```python
from build123d import *

# Parameters (mm, degrees)
BOSS_EXTRUDE1_DEPTH     = 5
CUT_EXTRUDE1_DEPTH      = 57
CUT_EXTRUDE1_DEPTH_BACK = 57
SKETCH2_R               = 3


with BuildPart() as part:
    # Sketch1 → Boss-Extrude1 (new body)
    with BuildSketch(Plane(origin=(0, 0, 0), x_dir=(1, 0, 0), z_dir=(0, 1, 0))):
        Polygon((0, -45), (21, -45), (21, -21), (45, -21), (45, 0), (295, 0), (295, -21), (319, -21), (319, -45), (340, -45), (340, -295), (319, -295), (319, -319), (295, -319), (295, -340), (45, -340), (45, -319), (21, -319), (21, -295), (0, -295), align=None)
    extrude(amount=BOSS_EXTRUDE1_DEPTH)

    # Sketch2 → Cut-Extrude1 (cut, two sides: drawn at the far end of the back side and taken through both)
    with BuildSketch(Plane(origin=(0, 5, 0), x_dir=(1, 0, 0), z_dir=(0, 1, 0)).offset(-CUT_EXTRUDE1_DEPTH_BACK)):
        with Locations(Location((100, -10, 0), (0, 0, 270))):
            Circle(SKETCH2_R)
        with Locations(Location((240, -10, 0), (0, 0, 270))):
            Circle(SKETCH2_R)
        with Locations(Location((240, -330, 0), (0, 0, 270))):
            Circle(SKETCH2_R)
        with Locations(Location((100, -330, 0), (0, 0, 270))):
            Circle(SKETCH2_R)
        with Locations(Location((10, -240, 0), (0, 0, 270))):
            Circle(SKETCH2_R)
        with Locations(Location((10, -100, 0), (0, 0, 270))):
            Circle(SKETCH2_R)
        with Locations(Location((330, -240, 0), (0, 0, 270))):
            Circle(SKETCH2_R)
        with Locations(Location((330, -100, 0), (0, 0, 270))):
            Circle(SKETCH2_R)
    extrude(amount=CUT_EXTRUDE1_DEPTH + CUT_EXTRUDE1_DEPTH_BACK, mode=Mode.SUBTRACT)


solid = part.part
```
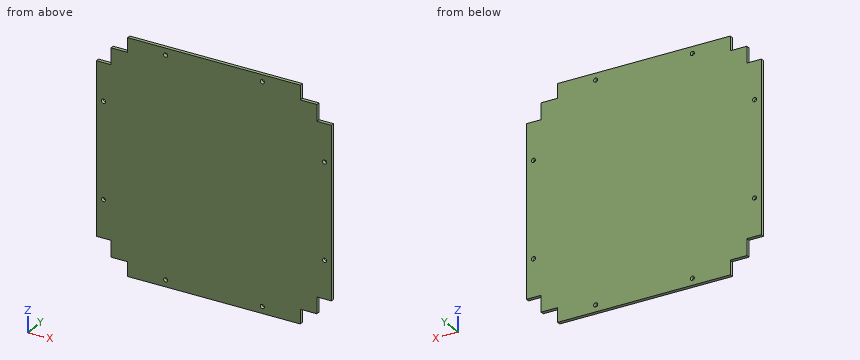
Source: CAD feature listing. Evaluate the final solid. Frame: model axes, mm. Round coordinates to 2 decimals unless told otherwise and drop trailing zeros. Write each loop counter-clockwise with the first axis right and the second up, starting at its lowest first coordinate (ties: lowest second). Pieces come first, ordered by that corner, then holes. Notation, with made-up numbers: M 1.25,0.25 L 43.25,0.25 A4 cw 43.25,7.25 Z; hole C 81,67 d10. An arc over 180 degrees is marked long. Answer as a JSON object with one key per item and string values. Group by question number.
(1) First-contact query: pin 1 (2.5 mm diameter, centred on x = 32, y = 3, fed in from +Z); pin 2 (2.5 mm diameter, centred on y = 3, z = 330, fed in from +X). Flat tips, straight axial feed; report the tip coordinate or a pass-through.
(2) Ray query, line 1 (X direction, y = 3.55, z = 330); line 2 (Z direction, x = 100, y = 1.2). Return the intervals inside material, ascending. Write a range as [from, to].
(3) Section query B-B on z = 32. Output: boundary loops of the cut face in (x, y), then the cut area to 3 significant figures.
(4) Section query A-A on y = 1.45. State how many separate pieces and enclosed holes the cut face has, then the cut area to 3 significant figures.
Computed values:
{
 "1": {"pin 1": "z = 319", "pin 2": "x = 295"},
 "2": {"line 1": "[45, 97], [103, 237], [243, 295]", "line 2": "[0, 7], [13, 327], [333, 340]"},
 "3": {"outline": "M 21,0 L 319,0 L 319,5 L 21,5 Z", "area": "1,490 mm^2"},
 "4": {"separate pieces": "1", "enclosed holes": "8", "area": "110,000 mm^2"}
}
